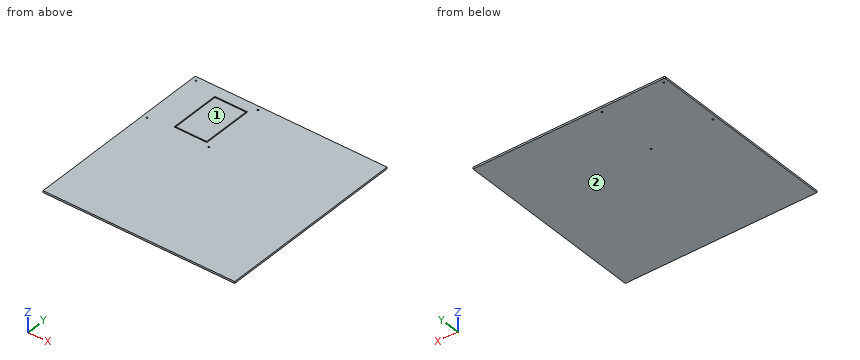
from build123d import *

# Parameters (mm, degrees)
ESQUISSE1_W        = 230
ESQUISSE1_H        = 230
ESQUISSE1_R        = 2.5
BOSS_EXTRU_1_DEPTH = 6
CONG_1_R           = 4
ESQUISSE2_W        = 106
ESQUISSE2_H        = 166
ESQUISSE2_W_2      = 102
ESQUISSE2_H_2      = 162
BOSS_EXTRU_2_DEPTH = 2
BOSS_EXTRU_3_DEPTH = 6


with BuildPart() as part:
    # Esquisse1 → Boss.-Extru.1 (new body)
    with BuildSketch(Plane.XY):
        with Locations((-28.150579015, -3.53164557)):
            Rectangle(ESQUISSE1_W, ESQUISSE1_H)
        with Locations((-129.150579015, 97.46835443)):
            Circle(ESQUISSE1_R, mode=Mode.SUBTRACT)
        with Locations((72.849420985, 97.46835443)):
            Circle(ESQUISSE1_R, mode=Mode.SUBTRACT)
        with Locations((72.849420985, -104.53164557)):
            Circle(ESQUISSE1_R, mode=Mode.SUBTRACT)
        with Locations((-129.150579015, -104.53164557)):
            Circle(ESQUISSE1_R, mode=Mode.SUBTRACT)
    extrude(amount=BOSS_EXTRU_1_DEPTH)

    # Congé1
    cong_1_edges = [part.edges().sort_by_distance(p)[0] for p in [
        (-143.150579015, 111.46835443, 3),
        (86.849420985, 111.46835443, 3),
        (86.849420985, -118.53164557, 3),
        (-143.150579015, -118.53164557, 3),
    ]]
    fillet(cong_1_edges, radius=CONG_1_R)

    # Esquisse2 → Boss.-Extru.2 (add)
    with BuildSketch(Plane.XY.offset(6)):
        with Locations((3.849420985, -9.53164557)):
            Rectangle(ESQUISSE2_W, ESQUISSE2_H)
        with Locations((3.849420985, -9.53164557)):
            Rectangle(ESQUISSE2_W_2, ESQUISSE2_H_2, mode=Mode.SUBTRACT)
    extrude(amount=BOSS_EXTRU_2_DEPTH)

    # Esquisse3 → Boss.-Extru.3 (add)
    with BuildSketch(Plane(origin=(0, 0, 0), x_dir=(-1, 0, 0), z_dir=(0, 0, -1))):
        Polygon((-82.849420985, 111.46835443), (-482.849420985, 111.46835443), (-482.849420985, -514.53164557), (143.150579015, -514.53164557), (143.150579015, -114.53164557), (-82.849420985, -114.53164557), align=None)
    extrude(amount=-BOSS_EXTRU_3_DEPTH)


solid = part.part
Read the model definition and answer for the solid it produces. Units are mm, in the model's axes. Face numbers are marked on the shaded views. Coordinates: 2 decimals unless noted, no trailing zeros. Loops run counter-clockwise (first coordinate to the right, second up) from the corner with the lowest first, then second, coordinate; pieces in that order, holes last.
Q1. The mould has two halves that part along Y. Classify the marked faces 1 and 2: +Y half, -Y half, draft (parallel to the pull), parting line (faces both ways), or undercut.
Q2. Each of these flat-tipped pins is pushed along its axis until it touches: pin 1 Ø4 at (x, y) = (72.85, -104.53) entering from +Z; pin 2 Ø1 at (y, z) = (-5, 7.5) entering from -X; pin 3 Ø1 at (x, z) = (1.5, 7) entering from -Y; pin 4 Ø0.6 at (y, z) = (30.5, 7) entering from +X. Where does it stop, or does it pass through?
Q3. The part is cut by section A-A on y = -51. Write down the section's boundary in (x, z), and give its area (3 significant figures).
Q4. Consider probe 1 along Z at (x, y) = (11, -311.5); probe 2 along X at (y, z) = (-64, 7.5). Determine where each line is inside the solid, lowest interval first.
Q5. The part is cut by section D-D on x = -58. Write down the section's boundary in (y, z), and give its area (3 significant figures).
Q6. The part is cut by section B-B on x = 27. Write down the section's boundary in (y, z), and give its area (3 significant figures).
Q7. The part is cut by section C-C on y = -280. Write down the section's boundary in (x, z), and give its area (3 significant figures).
Results below:
1. face 1: undercut
1. face 2: draft
2. pin 1: passes through
2. pin 2: stops at x = -49.15
2. pin 3: stops at y = -92.53
2. pin 4: stops at x = 56.85
3. outline: (-143.15, 0) - (482.85, 0) - (482.85, 6) - (56.85, 6) - (56.85, 8) - (54.85, 8) - (54.85, 6) - (-47.15, 6) - (-47.15, 8) - (-49.15, 8) - (-49.15, 6) - (-143.15, 6) - close
3. area: 3,760 mm2
4. probe 1: z = 0 to 6
4. probe 2: x = -49.15 to -47.15, 54.85 to 56.85
5. outline: (-514.53, 0) - (111.47, 0) - (111.47, 6) - (-514.53, 6) - close
5. area: 3,760 mm2
6. outline: (-514.53, 0) - (111.47, 0) - (111.47, 6) - (73.47, 6) - (73.47, 8) - (71.47, 8) - (71.47, 6) - (-90.53, 6) - (-90.53, 8) - (-92.53, 8) - (-92.53, 6) - (-514.53, 6) - close
6. area: 3,760 mm2
7. outline: (-143.15, 0) - (482.85, 0) - (482.85, 6) - (-143.15, 6) - close
7. area: 3,760 mm2
